Work out the finished part from the listing and answer in its coordinate system (mm). Give positions to 0.01 mm unless a question says otherwise; leave off trailing zeros. Order: outer loops, then holes, each group sorted by start corner. A loop starts at its lowest first (then second) coordinate and runs counter-clockwise, first axis right, second up.
Autodesk Inventor part; units mm, degrees
ref_plane "YZ Plane" through (0, 0, 0) normal (1, 0, 0) x (0, 1, 0)
ref_plane "XZ Plane" through (0, 0, 0) normal (0, 1, 0) x (-1, 0, 0)
ref_plane "XY Plane" through (0, 0, 0) normal (0, 0, 1) x (1, 0, 0)
sketch "Sketch1" plane through (0, 0, 0) normal (1, 0, 0) x (0, 1, 0)
  line L0 (-114.3, 300.99) -> (114.3, 300.99)
  line L1 (114.3, 300.99) -> (114.3, -300.99)
  line L2 (114.3, -300.99) -> (-114.3, -300.99)
  line L3 (-114.3, -300.99) -> (-114.3, 300.99)
  line L4 (-114.3, 300.99) -> (114.3, -300.99) construction
  line L5 (114.3, 300.99) -> (-114.3, -300.99) construction
  point P0 (0, 0)
  dimension "d3" = 228.6
  dimension "d4" = 601.98
extrude "Extrusion2" add sketch "Sketch1" along normal blind 2.8575
fillet "Fillet1" radius 10.16 4 edges at (1.4287, -114.3, -300.99) (1.4287, 114.3, -300.99) (1.4287, -114.3, 300.99) (1.4287, 114.3, 300.99)
fillet "Fillet2" radius 0.5715 16 edges at (2.8575, 111.3242, 298.0142) (2.8575, 0, 300.99) (2.8575, -111.3242, 298.0142) (2.8575, -114.3, 0) (2.8575, -111.3242, -298.0142) (2.8575, 0, -300.99) (2.8575, 111.3242, -298.0142) (2.8575, 114.3, 0) (0, 111.3242, -298.0142) (0, 0, -300.99) (0, -111.3242, -298.0142) (0, -114.3, 0) (0, -111.3242, 298.0142) (0, 0, 300.99) (0, 111.3242, 298.0142) (0, 114.3, 0)
sketch "Sketch3" plane through (0, 0, 0) normal (-1, 0, 0) x (0, 0, 1)
  line L0 (300.4185, 104.14) -> (300.4185, -104.14)
  line L1 (290.83, -113.7285) -> (-290.83, -113.7285)
  line L2 (-290.83, 113.7285) -> (290.83, 113.7285)
  line L3 (-300.4185, -104.14) -> (-300.4185, 104.14)
  line L4 (290.83, 113.7285) -> (-290.83, 113.7285)
  line L5 (-97.2185, 125.0999) -> (-97.2185, 80.4789)
  line L6 (-97.2185, 80.4789) -> (-198.8185, 80.4789)
  line L7 (-198.8185, 80.4789) -> (-198.8185, 125.0999)
  line L8 (-97.2185, 125.0999) -> (-198.8185, 125.0999)
  dimension "d48" = 101.6
  dimension "d49" = 101.6
  dimension "d50" = 0
  dimension "d63" = 11.3714
  dimension "d64" = 33.2496
extrude "Extrusion3" cut sketch "Sketch3" against normal blind 5.08
sketch "Sketch4" plane through (2.8575, 0, 0) normal (1, 0, 0) x (0, 0, -1)
  circle A0 centre (234.3785, 106.1085) radius 2.54
  circle A1 centre (262.3185, 106.1085) radius 2.54
  line L0 (-290.83, 113.7285) -> (290.83, 113.7285)
  line L1 (300.4185, 104.14) -> (300.4185, -104.14)
  circle A2 centre (-262.89, 106.1085) radius 2.54
  circle A3 centre (-234.95, 106.1085) radius 2.54
  line L2 (-300.99, 104.14) -> (-300.99, -104.14)
  point P0 (0, 0)
  point P1 (198.8185, 113.7285)
  dimension "d52" = 5.08
  dimension "d53" = 7.62
  dimension "d54" = 27.94
  dimension "d55" = 38.1
  dimension "d58" = 27.94
  dimension "d60" = 38.1
extrude "Extrusion5" cut sketch "Sketch4" against normal up to next
equation "\"d58\" = d54"
equation "\"d60\" = d55"
equation "\"d61\" = d54"
properties part number "SideFlap"
1. The part is cut by section A-A (x = 1.1). Write down the section's boundary in (y, z).
Findings below:
outline: (-114.3, -290.83) arc R10.16 ccw to (-104.14, -300.99) - (104.14, -300.99) arc R10.16 ccw to (114.3, -290.83) - (114.3, -198.82) - (80.48, -198.82) - (80.48, -97.22) - (114.3, -97.22) - (114.3, 290.83) arc R10.16 ccw to (104.14, 300.99) - (-104.14, 300.99) arc R10.16 ccw to (-114.3, 290.83) - close; hole circle Ø5.08 at (106.11, -262.32); hole circle Ø5.08 at (106.11, -234.38); hole circle Ø5.08 at (106.11, 234.95); hole circle Ø5.08 at (106.11, 262.89)
2. Given P1, Ø8, axis at y = 106.11, z = -262.32, coming from the +X side, flat-ended and moving along its own axis, determine where the tip first touches the part or whether it passes through.
Findings below:
P1: stops at x = 2.86
3. Straight lines are drawn through the part: probe 1 along Z at (x, y) = (0.25, 97.5); probe 2 along Y at (x, z) = (1.5, 262.89); probe 3 along Y at (x, z) = (1.55, -178). For each, find the intervals that lie inside material, in ascending order.
Findings below:
probe 1: z = -300.89 to -198.82, -97.22 to 300.89
probe 2: y = -114.3 to 103.57, 108.65 to 114.3
probe 3: y = -114.3 to 80.48
